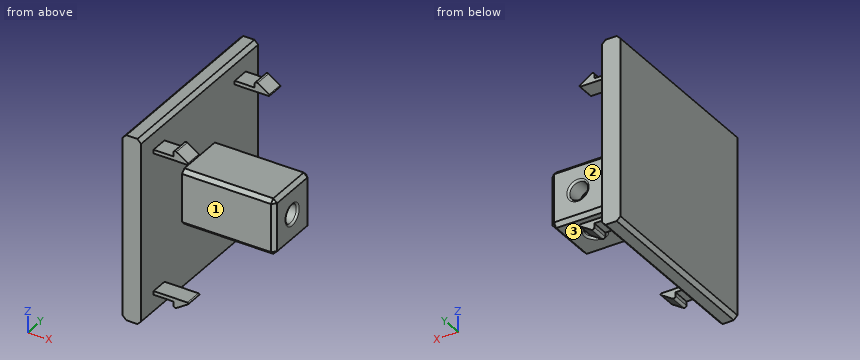
from build123d import *

# Parameters (mm, degrees)
BOSS_EXTRUDE2_DEPTH    = 50
CUT_EXTRUDE5_OUTLINE_W = 6.4
CUT_EXTRUDE5_OUTLINE_H = 5.3
CUT_EXTRUDE5_DEPTH     = 10
FILLET2_R              = 0.5
SKETCH33_W             = 15
SKETCH33_H             = 15
BOSS_EXTRUDE4_DEPTH    = 25
SKETCH34_R             = 2.5
CUT_EXTRUDE13_DEPTH    = 4.9
SKETCH37_R             = 2.5
CUT_EXTRUDE14_DEPTH    = 4.9
SKETCH38_R             = 2.5
CUT_EXTRUDE15_DEPTH    = 4.9
CHAMFER2_SIZE          = 1
FILLET3_R              = 0.5
CHAMFER3_SIZE          = 1
SKETCH40_W             = 10
SKETCH40_H             = 30
CUT_EXTRUDE17_DEPTH    = 76
FILLET4_R              = 0.25


# Read off the part's stored shape, not the designer's step: Cut-Extrude5
with BuildPart() as part:
    # Sketch3 → Boss-Extrude2 (new body)
    with BuildSketch(Plane(origin=(0, 0, 0), x_dir=(1, 0, 0), z_dir=(0, 1, 0))):
        Polygon((5, 44.6), (10.4, 44.6), (10.4, 46.6), (15, 43.6), (5, 43.6), (5, 6.4), (15, 6.4), (10.4, 3.4), (10.4, 5.4), (5, 5.4), (5, 0), (0, 0), (0, 50), (5, 50), align=None)
    extrude(amount=BOSS_EXTRUDE2_DEPTH)

    # Cut-Extrude5 outline → Cut-Extrude5 (cut)
    with BuildSketch(Plane(origin=(5, 0, 0), x_dir=(0, 0, -1), z_dir=(1, 0, 0))):
        with Locations((3.2, 2.65)):
            Rectangle(CUT_EXTRUDE5_OUTLINE_W, CUT_EXTRUDE5_OUTLINE_H)
        with Locations((3.2, 47.35)):
            Rectangle(CUT_EXTRUDE5_OUTLINE_W, CUT_EXTRUDE5_OUTLINE_H)
        with Locations((46.8, 2.65)):
            Rectangle(CUT_EXTRUDE5_OUTLINE_W, CUT_EXTRUDE5_OUTLINE_H)
        with Locations((46.8, 47.35)):
            Rectangle(CUT_EXTRUDE5_OUTLINE_W, CUT_EXTRUDE5_OUTLINE_H)
    extrude(amount=CUT_EXTRUDE5_DEPTH, mode=Mode.SUBTRACT)

    # Fillet2
    fillet2_edges = [part.edges().sort_by_distance(p)[0] for p in [
        (10.4, 25, -46.6),
        (10.4, 25, -3.4),
    ]]
    fillet(fillet2_edges, radius=FILLET2_R)

    # Sketch33 → Boss-Extrude4 (add)
    with BuildSketch(Plane(origin=(5, 0, 0), x_dir=(0, 0, -1), z_dir=(1, 0, 0))):
        with Locations((25, 25)):
            Rectangle(SKETCH33_W, SKETCH33_H)
    extrude(amount=BOSS_EXTRUDE4_DEPTH)

    # Sketch34 → Cut-Extrude13 (cut)
    with BuildSketch(Plane(origin=(0, 32.5, 0), x_dir=(1, 0, 0), z_dir=(0, 1, 0))):
        with Locations(Location((22.5, 25, 0), (0, 0, 270))):
            Circle(SKETCH34_R)
    extrude(amount=-CUT_EXTRUDE13_DEPTH, mode=Mode.SUBTRACT)

    # Sketch37 → Cut-Extrude14 (cut)
    with BuildSketch(Plane(origin=(30, 0, 0), x_dir=(0, 0, -1), z_dir=(1, 0, 0))):
        with Locations((25, 25)):
            Circle(SKETCH37_R)
    extrude(amount=-CUT_EXTRUDE14_DEPTH, mode=Mode.SUBTRACT)

    # Sketch38 → Cut-Extrude15 (cut)
    with BuildSketch(Plane(origin=(0, 0, -32.5), x_dir=(-1, 0, 0), z_dir=(0, 0, -1))):
        with Locations((-22.5, 25)):
            Circle(SKETCH38_R)
    extrude(amount=-CUT_EXTRUDE15_DEPTH, mode=Mode.SUBTRACT)

    # Chamfer2
    chamfer2_edges = [part.edges().sort_by_distance(p)[0] for p in [
        (17.5, 32.5, -17.5),
        (17.5, 17.5, -17.5),
        (17.5, 17.5, -32.5),
        (17.5, 32.5, -32.5),
        (30, 25, -17.5),
        (30, 17.5, -25),
        (30, 25, -32.5),
        (30, 32.5, -25),
    ]]
    chamfer(chamfer2_edges, length=CHAMFER2_SIZE)

    # Fillet3
    fillet3_edges = [part.edges().sort_by_distance(p)[0] for p in [
        (22.5, 32.5, -27.5),
        (30, 25, -22.5),
        (25, 25, -32.5),
    ]]
    fillet(fillet3_edges, radius=FILLET3_R)

    # Chamfer3
    chamfer3_edges = [part.edges().sort_by_distance(p)[0] for p in [
        (0, 25, 0),
        (0, 25, -50),
        (5, 25, -50),
        (5, 25, 0),
    ]]
    chamfer(chamfer3_edges, length=CHAMFER3_SIZE)

    # Sketch40 → Cut-Extrude17 (cut, through all)
    with BuildSketch(Plane(origin=(5, 0, 0), x_dir=(0, 0, -1), z_dir=(1, 0, 0))):
        with Locations((6, 25)):
            Rectangle(SKETCH40_W, SKETCH40_H)
        with Locations((44, 25)):
            Rectangle(SKETCH40_W, SKETCH40_H)
    extrude(amount=CUT_EXTRUDE17_DEPTH, mode=Mode.SUBTRACT)

    # Fillet4
    fillet4_edges = [part.edges().sort_by_distance(p)[0] for p in [
        (15, 7.65, -43.6),
        (15, 7.65, -6.4),
        (15, 42.35, -43.6),
        (15, 42.35, -6.4),
    ]]
    fillet(fillet4_edges, radius=FILLET4_R)


solid = part.part
Work out the finished part from the listing and answer in its coordinate system (mm). Face numbers are marked on the shaded views. A direction names the side the tool comes from. Give positions to 0.01 mm unless a question says otherwise; leave off trailing zeros. Write each loop counter-clockwise with the first axis right and the second up, starting at its lowest first coordinate (ties: lowest second). Pieces come first, ordered by that corner, then holes. Notation, with made-up numbers: (11.5, -27) - (59.5, -27) arc R24 cw to (59.5, -6) - close; hole circle Ø11 at (-38.5, 80). An arc over 180 degrees is marked (long way). One line per item, written item: value. Start each with the question number.
1. Find section D-D (y = 39). Write down the section's boundary in (x, z).
2. Find section A-A (y = 29). Write down the section's boundary in (x, z).
3. Consider probe 1 along Y at (x, z) = (11, -6); probe 2 along X at (y, z) = (30.05, -25); probe 3 along Y at (x, z) = (27, -25). Determine where each line is inside the solid, lowest interval first.
4. Find section C-C (x = 28). Write down the section's boundary in (y, z), then the cut area to 3 significant figures.
5. Find section B-B (x = 9). Write down the section's boundary in (y, z).
6. For the marked faces 1, 2 and 3, determine the directions among +Z, -Z, +X, -X, +Y, -Y from which every point of the face is accessible in a straight line to the end or side of a thin tool.
7. Given pin 1 (1.3 mm diameter, centred on x = 11, z = -44.5, fed in from +Y); pin 2 (4.5 mm diameter, centred on x = 22.5, z = -25, fed in from -Y); pin 3 (2.5 mm diameter, centred on x = 6.5, y = 42, fed in from +Z); pin 4 (5.5 mm diameter, centred on y = 26, z = -26, fed in from +X), each flat-ended and moving along its own axis, determine where each tip first touches the part or whether it passes through.
Geometry results:
1. outline: (0, -49) - (1, -50) - (4, -50) - (5, -49) - (5, -1) - (4, 0) - (1, 0) - (0, -1) - close
2. outline: (0, -49) - (1, -50) - (4, -50) - (5, -49) - (5, -32.5) - (29, -32.5) - (30, -31.5) - (30, -18.5) - (29, -17.5) - (5, -17.5) - (5, -1) - (4, 0) - (1, 0) - (0, -1) - close; hole circle Ø5 at (22.5, -25)
3. probe 1: 5.3 to 10, 40 to 44.7
3. probe 2: 0 to 20, 25 to 30
3. probe 3: 17.5 to 22.5, 27.5 to 32.5
4. outline: (17.5, -31.5) - (18.5, -32.5) - (31.5, -32.5) - (32.5, -31.5) - (32.5, -18.5) - (31.5, -17.5) - (18.5, -17.5) - (17.5, -18.5) - close; hole circle Ø5 at (25, -25)
4. area: 203 mm2
5. outline: (5.3, -44.6) - (10, -44.6) - (10, -43.6) - (5.3, -43.6) - close; (5.3, -6.4) - (10, -6.4) - (10, -5.4) - (5.3, -5.4) - close; (17.5, -31.5) - (18.5, -32.5) - (31.5, -32.5) - (32.5, -31.5) - (32.5, -18.5) - (31.5, -17.5) - (18.5, -17.5) - (17.5, -18.5) - close; (40, -44.6) - (44.7, -44.6) - (44.7, -43.6) - (40, -43.6) - close; (40, -6.4) - (44.7, -6.4) - (44.7, -5.4) - (40, -5.4) - close
6. face 1: +Z, -Z, +X, -Y
6. face 2: +Z, -Z, +X, +Y
6. face 3: -Z, +X, +Y, -Y
7. pin 1: y = 44.7
7. pin 2: y = 17.5
7. pin 3: z = -5.4
7. pin 4: x = 30
